Check sheet for the modelled part. Datum: model origin and axes. Units: mm. Face numbers are marked on the shaded views. A direction names the side the tool comes from. Coordinates: 2 decimals unless noted, no trailing zeros. Loops run counter-clockwise (first coordinate to the right, second up) from the corner with the lowest first, then second, coordinate; pieces in that order, holes last. Notation, with made-up numbers: (40, 16) - (56, 16) arc R31 cw to (56, 43) - close; hole circle Ø3 at (-16.5, 25.5). An arc over 180 degrees is marked (long way). Use a Markdown table: item, result. Add a question column.
1) Thickness scan on line 1 (X direction, y = 50.8, z = -21.5); line 2 (Y direction, x = -50.8, z = -20); line 3 (Z direction, x = -10, y = 30.5). Record the ranges inside material, lowest first.
2) Go/stop test with flat-tipped pins: P1, Ø23, axis at x = -0.5, y = -11, coming from the +Z side; P2, Ø11.5, axis at x = -50.8, y = 50.8, coming from the -Z side. Record where each tip stops, or that it passes through.
3) Tool access check on the marked faces 1 and 2. Record the directions out of +Z, -Z, +X, -X, +Y, -Y that give a thin tool (end or side, any length) a straight path to the whole face; none if there is none.
4) Sectioned sample at A-A, the plane z = -15. Enter the section's corners in (x, y).
5) Draft check along X on the marked faces 3, 4 and 5. Enter one of: pulls with the +X half, pulls with the -X half, needs draft (parallel to the pull), parting line crosses it, or undercut.
6) Sectioned sample at B-B, the plane x = 0. Enter the section's corners in (y, z), then the cut area to 3 significant figures.
from build123d import *

# Parameters (mm, degrees)
F2_DEPTH = 63.5
F5_DEPTH = 50.8
F7_DEPTH = 50.8


with BuildPart() as f2:
    # F1 (on Front) → F2 (new body, symmetric)
    with BuildSketch(Plane.XZ):
        Polygon((-63.5, -32.291652), (63.5, -32.291652), (63.5, 5.808348), (0, 5.808348), (-63.5, 5.808348), align=None)
    extrude(amount=F2_DEPTH, both=True)

    # F0 (on Front) → F3 (revolve, cut)
    with BuildSketch(Plane.XZ):
        Polygon((38.1, -1.524), (50.8, 5.808348), (0, 5.808348), (0, -1.524), align=None)
    revolve(axis=Axis((0, 0, 2.142174), (0, 0, -1)), mode=Mode.SUBTRACT)

    # F4 (on Top) → F5 (cut, symmetric)
    with BuildSketch(Plane.XY):
        with BuildLine():
            ThreePointArc((-44.45, 50.8), (-55.290128, 55.290128), (-50.8, 44.45))
            Line((-50.8, 44.45), (-50.8, 50.8))
            Line((-50.8, 50.8), (-44.45, 50.8))
        make_face()
        with BuildLine():
            Line((-50.8, 50.8), (-50.8, 44.45))
            ThreePointArc((-50.8, 44.45), (-46.309872, 46.309872), (-44.45, 50.8))
            Line((-44.45, 50.8), (-50.8, 50.8))
        make_face()
    extrude(amount=F5_DEPTH, both=True, mode=Mode.SUBTRACT)

    # F6 (on Top) → F7 (cut, symmetric)
    with BuildSketch(Plane.XY):
        with BuildLine():
            ThreePointArc((50.8, -44.45), (46.309872, -46.309872), (44.45, -50.8))
            Line((44.45, -50.8), (50.8, -50.8))
            Line((50.8, -50.8), (50.8, -44.45))
        make_face()
        with BuildLine():
            Line((50.8, -50.8), (44.45, -50.8))
            ThreePointArc((44.45, -50.8), (50.8, -57.15), (57.15, -50.8))
            ThreePointArc((57.15, -50.8), (55.290128, -46.309872), (50.8, -44.45))
            Line((50.8, -44.45), (50.8, -50.8))
        make_face()
    extrude(amount=F7_DEPTH, both=True, mode=Mode.SUBTRACT)


solid = f2.part
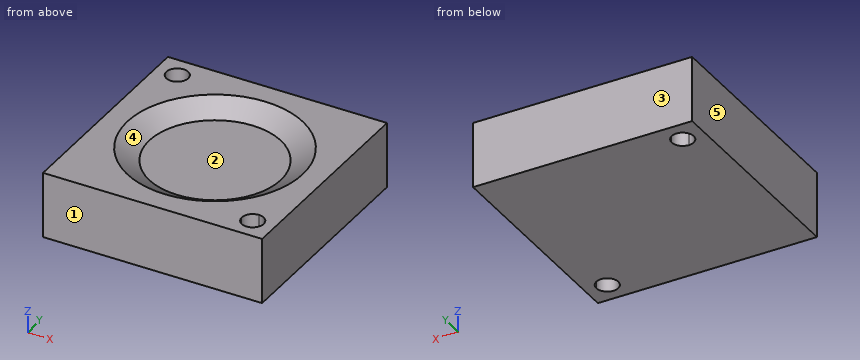
Solved:
| question | item | result |
|---|---|---|
| 1 | line 1 | x = -63.5 to -57.15, -44.45 to 63.5 |
| 1 | line 2 | y = -63.5 to 44.45, 57.15 to 63.5 |
| 1 | line 3 | z = -32.29 to -1.52 |
| 2 | P1 | stops at z = -1.52 |
| 2 | P2 | passes through |
| 3 | face 1 | +Z, -Z, +X, -X, -Y |
| 3 | face 2 | +Z |
| 4 | outline | (-63.5, -63.5) - (63.5, -63.5) - (63.5, 63.5) - (-63.5, 63.5) - close; hole circle Ø12.7 at (-50.8, 50.8); hole circle Ø12.7 at (50.8, -50.8) |
| 5 | face 3 | needs draft |
| 5 | face 4 | undercut |
| 5 | face 5 | pulls with the -X half |
| 6 | outline | (-63.5, -32.29) - (63.5, -32.29) - (63.5, 5.81) - (50.8, 5.81) - (38.1, -1.52) - (-38.1, -1.52) - (-50.8, 5.81) - (-63.5, 5.81) - close |
| 6 | area | 4,190 mm2 |
